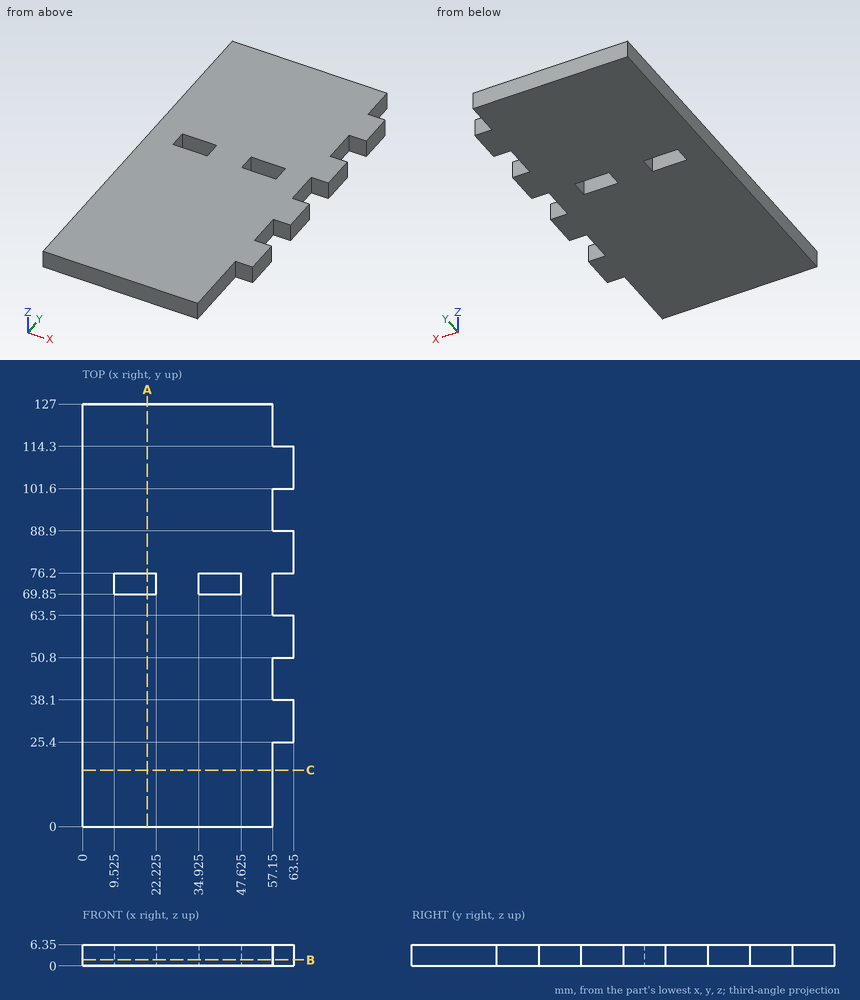
Design review of the part shown in the three views and the two pictorial views. Dimensions are in mm from the part's minimum x, y and z. Round coordinates to 2 decimals unless told otherwise and drop trailing zeros. Order: outer loops, then holes, each group sorted by start corner. A loop starts at its lowest first (then second) coordinate and runs counter-clockwise, first axis right, second up. Notation, with made-up numbers: (11.25, 28) - (27.25, 28) arc R19 ccw to (27.25, 53) - close; hole circle Ø5 at (-26, 25.5). An arc over 180 degrees is marked (long way). One line per question, with ' | ' between items.
Item 1: For P1, Ø3, axis at x = 60, z = 3, coming from the -Y side; P2, Ø1.9, axis at y = 70.5, z = 3, coming from the +X side; P3, Ø1.9, axis at x = 60, z = 3, coming from the +Y side, all flat-tipped, find the tip position at first contact; note any pin that passes through.
Checks:
P1: y = 25.4 | P2: x = 57.15 | P3: y = 114.3
Item 2: Take a section at C-C, the plane y = 17. Write out the cut boundary in (x, z).
Checks:
outline: (0, 0) - (57.15, 0) - (57.15, 6.35) - (0, 6.35) - close
Item 3: Wall thickness on line 1 (Y direction, x = 59, z = 4.25); line 2 (Y direction, x = 10, z = 4.25); line 3 (X direction, y = 72, z = 5) (3 decimals): over which ranges is each line inside the solid? List them lowest first. Write a range as [from, to].
Checks:
line 1: [25.4, 38.1], [50.8, 63.5], [76.2, 88.9], [101.6, 114.3] | line 2: [0, 69.85], [76.2, 127] | line 3: [0, 9.525], [22.225, 34.925], [47.625, 57.15]
Item 4: Take a section at B-B, the plane z = 1.75. Write out the cut boundary in (x, y) (3 decimals), then the cut area to 3 significant figures.
Checks:
outline: (0, 0) - (57.15, 0) - (57.15, 25.4) - (63.5, 25.4) - (63.5, 38.1) - (57.15, 38.1) - (57.15, 50.8) - (63.5, 50.8) - (63.5, 63.5) - (57.15, 63.5) - (57.15, 76.2) - (63.5, 76.2) - (63.5, 88.9) - (57.15, 88.9) - (57.15, 101.6) - (63.5, 101.6) - (63.5, 114.3) - (57.15, 114.3) - (57.15, 127) - (0, 127) - close; hole (9.525, 69.85) - (22.225, 69.85) - (22.225, 76.2) - (9.525, 76.2) - close; hole (34.925, 69.85) - (47.625, 69.85) - (47.625, 76.2) - (34.925, 76.2) - close | area: 7,420 mm²
Item 5: Take a section at A-A, the plane x = 19.5. Write out the cut boundary in (y, z), then the cut area to 3 significant figures.
Checks:
outline: (0, 0) - (69.85, 0) - (69.85, 6.35) - (0, 6.35) - close; (76.2, 0) - (127, 0) - (127, 6.35) - (76.2, 6.35) - close | area: 766 mm²
